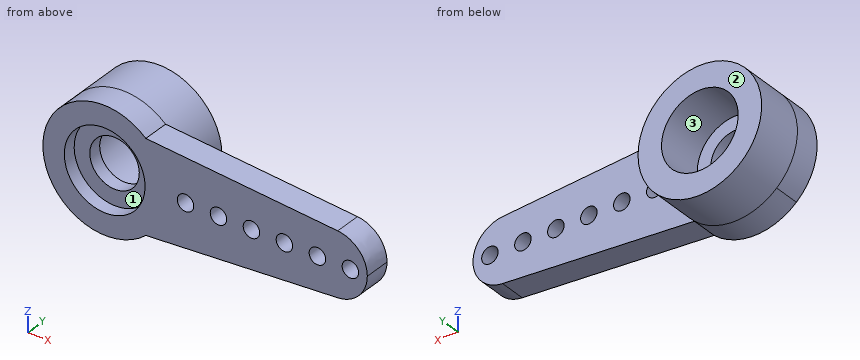
from build123d import *

# Parameters (mm, degrees)
SKETCH1_R               = 0.5
SKETCH1_R_2             = 1.5
BOSS_EXTRUDE1_DEPTH     = 1.6
SKETCH2_R               = 3.75
SKETCH2_R_2             = 2.325
BOSS_EXTRUDE2_DEPTH     = 2.9
FILLET1_START           = -1
FILLET1_DEPTH           = 4
FILLET2_START           = -1
FILLET2_DEPTH           = 4
SKETCH3_R               = 2.45
CUT_EXTRUDE1_DEPTH      = 0.8
ENL_V_START             = -10
ENL_V_MAT_EXTRU_1_DEPTH = 10


with BuildPart() as part:
    # Sketch1 → Boss-Extrude1 (new body)
    with BuildSketch(Plane(origin=(0, 0, 0), x_dir=(1, 0, 0), z_dir=(0, 1, 0))):
        with BuildLine():
            Line((2.494493937, 2.8), (14.9, 1.875))
            ThreePointArc((14.9, 1.875), (15.925, 0), (14.9, -1.875))
            Line((14.9, -1.875), (2.494493937, -2.8))
            ThreePointArc((2.494493937, -2.8), (0, -3.75), (-2.494493937, -2.8))
            Line((-2.494493937, -2.8), (-14.9, -1.875))
            ThreePointArc((-14.9, -1.875), (-15.925, 0), (-14.9, 1.875))
            Line((-14.9, 1.875), (-2.494493937, 2.8))
            ThreePointArc((-2.494493937, 2.8), (0, 3.75), (2.494493937, 2.8))
        make_face()
        with Locations(Location((4.9, 0, 0), (0, 0, 270))):
            Circle(SKETCH1_R, mode=Mode.SUBTRACT)
        with Locations(Location((6.9, 0, 0), (0, 0, 270))):
            Circle(SKETCH1_R, mode=Mode.SUBTRACT)
        with Locations(Location((8.9, 0, 0), (0, 0, 270))):
            Circle(SKETCH1_R, mode=Mode.SUBTRACT)
        with Locations(Location((10.9, 0, 0), (0, 0, 270))):
            Circle(SKETCH1_R, mode=Mode.SUBTRACT)
        with Locations(Location((12.9, 0, 0), (0, 0, 270))):
            Circle(SKETCH1_R, mode=Mode.SUBTRACT)
        with Locations(Location((14.9, 0, 0), (0, 0, 270))):
            Circle(SKETCH1_R, mode=Mode.SUBTRACT)
        with Locations(Location((-14.9, 0, 0), (0, 0, 90))):
            Circle(SKETCH1_R, mode=Mode.SUBTRACT)
        with Locations(Location((-12.9, 0, 0), (0, 0, 90))):
            Circle(SKETCH1_R, mode=Mode.SUBTRACT)
        with Locations(Location((-10.9, 0, 0), (0, 0, 90))):
            Circle(SKETCH1_R, mode=Mode.SUBTRACT)
        with Locations(Location((-8.9, 0, 0), (0, 0, 90))):
            Circle(SKETCH1_R, mode=Mode.SUBTRACT)
        with Locations(Location((-6.9, 0, 0), (0, 0, 90))):
            Circle(SKETCH1_R, mode=Mode.SUBTRACT)
        with Locations(Location((-4.9, 0, 0), (0, 0, 90))):
            Circle(SKETCH1_R, mode=Mode.SUBTRACT)
        with Locations(Location((0, 0, 0), (0, 0, 270))):
            Circle(SKETCH1_R_2, mode=Mode.SUBTRACT)
    extrude(amount=BOSS_EXTRUDE1_DEPTH)

    # Sketch2 → Boss-Extrude2 (add)
    with BuildSketch(Plane(origin=(0, 1.6, 0), x_dir=(1, 0, 0), z_dir=(0, 1, 0))):
        with Locations(Location((0, 0, 0), (0, 0, 48.302453397))):
            Circle(SKETCH2_R)
        with Locations(Location((0, 0, 0), (0, 0, 270))):
            Circle(SKETCH2_R_2, mode=Mode.SUBTRACT)
    extrude(amount=BOSS_EXTRUDE2_DEPTH)

    # Fillet1: read off the stored shape, not the designer's step
    # Fillet1 outline → Fillet1 (cut)
    with BuildSketch(Plane(origin=(0, 0, 0), x_dir=(1, 0, 0), z_dir=(0, 1, 0)).offset(FILLET1_START)):
        with BuildLine():
            Line((-14.9, -1.875), (-14.131406802, -1.932309126))
            add(Edge.make_bspline(
                [(-14.131406802, -1.932309126), (-15.060349902, -1.863043724), (-15.925, -1.199048162), (-15.925, 0)],
                knots=[0, 0, 0, 0, 0.5, 0.5, 0.5, 0.5], degree=3, weights=[1, 0.691452416, 0.537178624, 0.537178624]))
            ThreePointArc((-15.925, 0), (-15.652023077, -1.068439282), (-14.9, -1.875))
        make_face()
        with BuildLine():
            ThreePointArc((-14.9, 1.875), (-15.652023077, 1.068439282), (-15.925, 0))
            add(Edge.make_bspline(
                [(-15.925, 0), (-15.925, 1.199048162), (-15.060349902, 1.863043724), (-14.131406802, 1.932309126)],
                knots=[0.5, 0.5, 0.5, 0.5, 1, 1, 1, 1], degree=3, weights=[0.537178624, 0.537178624, 0.691452416, 1]))
            Line((-14.131406802, 1.932309126), (-14.9, 1.875))
        make_face()
    extrude(amount=FILLET1_DEPTH, mode=Mode.SUBTRACT)

    # Fillet2: read off the stored shape, not the designer's step
    # Fillet2 outline → Fillet2 (cut)
    with BuildSketch(Plane(origin=(0, 0, 0), x_dir=(1, 0, 0), z_dir=(0, 1, 0)).offset(FILLET2_START)):
        with BuildLine():
            Line((14.9, 1.875), (14.131406802, 1.932309126))
            add(Edge.make_bspline(
                [(14.131406802, 1.932309126), (15.060349902, 1.863043724), (15.925, 1.199048162), (15.925, 0)],
                knots=[0, 0, 0, 0, 0.5, 0.5, 0.5, 0.5], degree=3, weights=[1, 0.691452416, 0.537178624, 0.537178624]))
            ThreePointArc((15.925, 0), (15.652023077, 1.068439282), (14.9, 1.875))
        make_face()
        with BuildLine():
            ThreePointArc((14.9, -1.875), (15.652023077, -1.068439282), (15.925, 0))
            add(Edge.make_bspline(
                [(15.925, 0), (15.925, -1.199048162), (15.060349902, -1.863043724), (14.131406802, -1.932309126)],
                knots=[0.5, 0.5, 0.5, 0.5, 1, 1, 1, 1], degree=3, weights=[0.537178624, 0.537178624, 0.691452416, 1]))
            Line((14.131406802, -1.932309126), (14.9, -1.875))
        make_face()
    extrude(amount=FILLET2_DEPTH, mode=Mode.SUBTRACT)

    # Sketch3 → Cut-Extrude1 (cut)
    with BuildSketch(Plane.XZ):
        with Locations(Location((0, 0, 0), (0, 0, 270))):
            Circle(SKETCH3_R)
    extrude(amount=-CUT_EXTRUDE1_DEPTH, mode=Mode.SUBTRACT)

    # Esquisse1 → Enlèv. mat.-Extru.1 (cut)
    with BuildSketch(Plane(origin=(0, 1.6, 0), x_dir=(1, 0, 0), z_dir=(0, 1, 0)).offset(ENL_V_START)):
        with BuildLine():
            Line((-2.494493937, 2.8), (-5.326259476, 9.645712634))
            Line((-5.326259476, 9.645712634), (-26.688602042, 9.645712634))
            Line((-26.688602042, 9.645712634), (-23.449621421, -3.244588312))
            Line((-23.449621421, -3.244588312), (-9.542304725, -12.289889455))
            Line((-9.542304725, -12.289889455), (-2.045012757, -5.407049631))
            Line((-2.045012757, -5.407049631), (-2.494493937, -2.8))
            ThreePointArc((-2.494493937, -2.8), (-3.75, 0), (-2.494493937, 2.8))
        make_face()
    extrude(amount=ENL_V_MAT_EXTRU_1_DEPTH, mode=Mode.SUBTRACT)


solid = part.part
CAD build for the part. Positions are in the model's coordinates, mm. Face numbers are marked on the shaded views. A direction names the side the tool comes from. Round coordinates to 2 decimals unless told otherwise and drop trailing zeros. Order: outer loops, then holes, each group sorted by start corner. A loop starts at its lowest first (then second) coordinate and runs counter-clockwise, first axis right, second up. Notation, with made-up numbers: M 11,-26 L 64,-26 A32 ccw 64,0 Z; hole C 24.25,34 d3. An arc over 180 degrees is marked long. Use one line per item in the form item = value.
Q1. Saw through at D-D on z = -0.25. State how many separate pieces and enclosed holes the cut face has, then the cut area to 3 significant figures.
Recorded:
separate_pieces = 8
enclosed_holes = 0
area = 25.2 mm^2
Q2. Which spindle directions (+Z, -Z, +X, -X, +Y, -Y) get a long thin tool onto all of the face, cutting with end or side? Do the marked faces 1, 2 and 3. Say none if no direction does.
Recorded:
face_1 = -Y
face_2 = +Z, -Z, +X, -X, +Y
face_3 = +Y
Q3. Saw through at A-A on x = 0. Give the cut face in (y, z) (3 decimals).
Recorded:
outline = M 0,-3.75 L 4.5,-3.75 L 4.5,-2.325 L 1.6,-2.325 L 1.6,-1.5 L 0.8,-1.5 L 0.8,-2.45 L 0,-2.45 Z; M 0,2.45 L 0.8,2.45 L 0.8,1.5 L 1.6,1.5 L 1.6,2.325 L 4.5,2.325 L 4.5,3.75 L 0,3.75 Z
Q4. Flat gauge pins, fed straight in: P1, Ø1.5, axis at x = 1, y = 2.5, coming from the -Z side; P2, Ø1.5, axis at y = 2.5, z = 0.5, coming from the +X side; P3, Ø1.8, axis at x = 0, z = 0, coming from the +Y side; P4, Ø3, axis at x = 7.5, z = 0.5, coming from the +Y side. Where does each tip first touch, or does it go through?
Recorded:
P1 = -3.74
P2 = 3.75
P3 = through
P4 = 1.6
Q5. Probe L1, parallel to Z at x = 0, y = 1.15; L2, parallel to X at y = 2.6, z = -1.75; L3, parallel to Y at x = 6, z = 0.5. List the from-to ranges inside material, lowest first.
Recorded:
L1 = -3.75 to -1.5, 1.5 to 3.75
L2 = -3.32 to -1.53, 1.53 to 3.32
L3 = 0 to 1.6
Q6. Saw through at C-C on x = 12.9. Give the cut face in (y, z).
Recorded:
outline = M 0,-2.02 L 1.6,-2.02 L 1.6,-0.5 L 0,-0.5 Z; M 0,0.5 L 1.6,0.5 L 1.6,2.02 L 0,2.02 Z
